Here's the drawing with two shaded views (mm, measured from the low corner). I have some questions. Coordinates: 2 decimals unless noted, no trailing zeros. Loops run counter-clockwise (first coordinate to the right, second up) from the corner with the lowest first, then second, coordinate; pieces in that order, holes last.
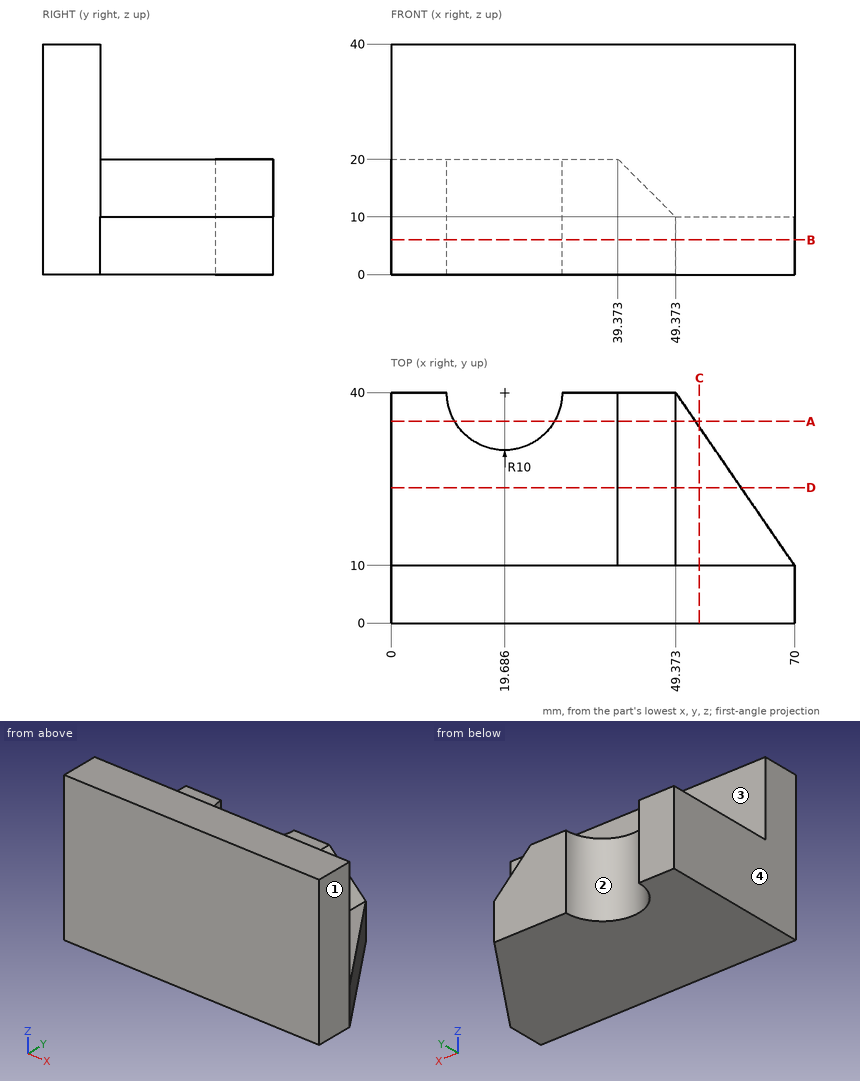
Q1. We'd pull the mould along X, two halves only. Please class the marked faces 1, 2, 3 and 4: pulls with the +X half, pulls with the -X half, needs draft (parallel to the pull), parting line crosses it, or undercut.
Q2. Suppose I cut it at A-A on y = 35. Write out the boundary of the cut face in (x, z).
Q3. Suppose I cut it at D-D on y = 23.5. Write out the boundary of the cut face in (x, z), and give its area (3 significant figures).
Q4. Suppose I cut it at B-B on z = 6. Write out the boundary of the cut face in (x, y), and give its area (3 significant figures).
Q5. Suppose I cut it at C-C on x = 53.5. Write out the boundary of the cut face in (y, z).
Q6. Please list where these lines run through material, in increasing order: probe 1 along Y at (x, z) = (39, 30.5); probe 2 along Z at (x, y) = (24.5, 12).
Q7. Will these pins go through, and if not, where does the flat tip stop? P1, Ø6, axis at x = 28.5, z = 36, coming from the +Y side; P2, Ø6, axis at x = 58, y = 27, coming from the +Z side; P3, Ø6, axis at x = 49, y = 15, coming from the +Z side.
Check values:
1. face 1: pulls with the +X half
1. face 2: undercut
1. face 3: needs draft
1. face 4: pulls with the -X half
2. outline: (0, 0) - (11.03, 0) - (11.03, 20) - (0, 20) - close; (28.35, 0) - (52.81, 0) - (52.81, 10) - (49.37, 10) - (39.37, 20) - (28.35, 20) - close
3. outline: (0, 0) - (60.72, 0) - (60.72, 10) - (49.37, 10) - (39.37, 20) - (0, 20) - close
3. area: 1,050 mm2
4. outline: (0, 0) - (70, 0) - (70, 10) - (49.37, 40) - (29.69, 40) arc R10 cw to (9.69, 40) - (0, 40) - close
4. area: 2,330 mm2
5. outline: (0, 0) - (34, 0) - (34, 10) - (10, 10) - (10, 40) - (0, 40) - close
6. probe 1: y = 0 to 10
6. probe 2: z = 0 to 20
7. P1: stops at y = 10
7. P2: stops at z = 10
7. P3: stops at z = 13.37
